Geometry: see drawing. Coordinates: mm, zero at the bounding-box minimum. Round coordinates to 2 decimals unless told otherwise and drop trailing zeros. Write each loop counter-clockwise with the first axis right and the second up, starting at its lowest first coordinate (ties: lowest second). Pieces come first, ordered by that corner, then holes. Notation, with made-up numbers: (-24, 54.5) -> (-11, 54.5) arc R27 cw to (-11, 75.5) -> close; hole circle Ø7 at (10, 17.25). An arc over 180 degrees is marked (long way). Write item = value, one per line. Start each with the question number.
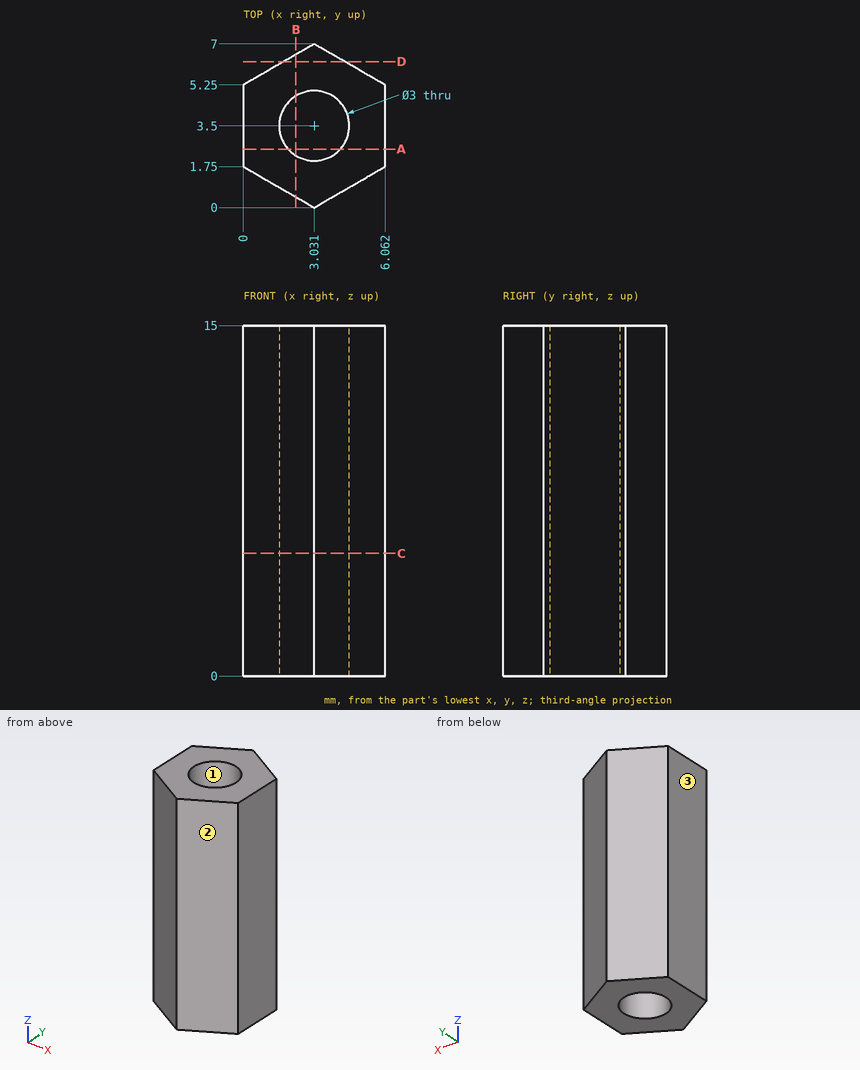
1. Pin query (flat end, axial travel): P1, Ø3, axis at y = 1.5, z = 6.5, coming from the +X side; P2, Ø1, axis at y = 6, z = 8, coming from the +X side. Return the tip coordinate at first contact, or that it passes through.
2. Section B-B (x = 2.25). Output: boundary loops of the cut face in (y, z).
3. Section A-A (y = 2.5). Output: boundary loops of the cut face in (x, z), then the cut area to 3 significant figures.
4. Section D-D (y = 6.25). Output: boundary loops of the cut face in (x, z).
5. Section C-C (z = 5.25). Output: boundary loops of the cut face in (x, y).
6. Line query: line 1 along Y through (x, z) = (1.75, 7.5); line 2 along Y through (x, z) = (4, 8.5) (1 decimal); line 3 along X through (y, z) = (4, 13.75) (1 decimal). Output: solid intervals per line, ascending.
7. Mould query, pull axis Y, two halves, no side actions, for the marked faces 1, 2 and 3. Classes: pulls with the +Y half, pulls with the -Y half, needs draft (parallel to the pull), parting line crosses it, or undercut.
Check sheet entries:
q1.P1 = 6.06
q1.P2 = 5.63
q2.outline = (0.45, 0) -> (2.22, 0) -> (2.22, 15) -> (0.45, 15) -> close; (4.78, 0) -> (6.55, 0) -> (6.55, 15) -> (4.78, 15) -> close
q3.outline = (0, 0) -> (1.91, 0) -> (1.91, 15) -> (0, 15) -> close; (4.15, 0) -> (6.06, 0) -> (6.06, 15) -> (4.15, 15) -> close
q3.area = 57.4 mm2
q4.outline = (1.73, 0) -> (4.33, 0) -> (4.33, 15) -> (1.73, 15) -> close
q5.outline = (0, 1.75) -> (3.03, 0) -> (6.06, 1.75) -> (6.06, 5.25) -> (3.03, 7) -> (0, 5.25) -> close; hole circle Ø3 at (3.03, 3.5)
q6.line_1 = 0.74 to 2.72, 4.28 to 6.26
q6.line_2 = 0.6 to 2.4, 4.6 to 6.4
q6.line_3 = 0 to 1.6, 4.4 to 6.1
q7.face_1 = undercut
q7.face_2 = pulls with the -Y half
q7.face_3 = needs draft
